```python
from build123d import *

# Parameters (mm, degrees)
SKETCH_2_W          = 1055.327979506
SKETCH_2_H          = 140
SKETCH_2_R          = 3
SKETCH_2_R_2        = 2.999999994
SKETCH_2_R_3        = 3.000000004
SKETCH_2_R_4        = 3.000000008
SKETCH_2_R_5        = 2.984817456
EXTRUDE_1_DEPTH     = 80
SKETCH_3_R          = 3
SKETCH_3_R_2        = 3.000000003
SKETCH_3_R_3        = 2.999999996
CUT_EXTRUDE_1_DEPTH = 10


with BuildPart() as part:
    # Эскиз2 → Бобышка-Вытянуть1 (new body)
    with BuildSketch(Plane(origin=(35, -236.577126762, 8.404450588), x_dir=(-1.3965925355372533e-14, -0.44721359549995804, -0.8944271909999159), z_dir=(2.4440369371901933e-14, -0.8944271909999159, 0.44721359549995804))):
        with Locations((247.509812295, 0)):
            Rectangle(SKETCH_2_W, SKETCH_2_H)
        with Locations((-220.154177458, 48.999999999)):
            Circle(SKETCH_2_R, mode=Mode.SUBTRACT)
        with Locations((-130.154177458, 49)):
            Circle(SKETCH_2_R, mode=Mode.SUBTRACT)
        with Locations((-220.154177458, -41.000000001)):
            Circle(SKETCH_2_R, mode=Mode.SUBTRACT)
        with Locations((-130.154177458, -41)):
            Circle(SKETCH_2_R, mode=Mode.SUBTRACT)
        with Locations((-40, 50)):
            Circle(SKETCH_2_R, mode=Mode.SUBTRACT)
        with Locations((-40, -40)):
            Circle(SKETCH_2_R, mode=Mode.SUBTRACT)
        with Locations((50, 50)):
            Circle(SKETCH_2_R, mode=Mode.SUBTRACT)
        with Locations((50, -40)):
            Circle(SKETCH_2_R, mode=Mode.SUBTRACT)
        with Locations((75, 50)):
            Circle(SKETCH_2_R, mode=Mode.SUBTRACT)
        with Locations((75, -40)):
            Circle(SKETCH_2_R, mode=Mode.SUBTRACT)
        with Locations((105, -57.5)):
            Circle(SKETCH_2_R, mode=Mode.SUBTRACT)
        with Locations((105, 35.5)):
            Circle(SKETCH_2_R, mode=Mode.SUBTRACT)
        with Locations((210, -57.5)):
            Circle(SKETCH_2_R, mode=Mode.SUBTRACT)
        with Locations((210, 35.5)):
            Circle(SKETCH_2_R, mode=Mode.SUBTRACT)
        with Locations((280, 50)):
            Circle(SKETCH_2_R, mode=Mode.SUBTRACT)
        with Locations((280, -41)):
            Circle(SKETCH_2_R, mode=Mode.SUBTRACT)
        with Locations((420, 50)):
            Circle(SKETCH_2_R, mode=Mode.SUBTRACT)
        with Locations((420, -40)):
            Circle(SKETCH_2_R, mode=Mode.SUBTRACT)
        with Locations((445, 50)):
            Circle(SKETCH_2_R, mode=Mode.SUBTRACT)
        with Locations((445, -40)):
            Circle(SKETCH_2_R, mode=Mode.SUBTRACT)
        with Locations((535, 50)):
            Circle(SKETCH_2_R, mode=Mode.SUBTRACT)
        with Locations((535, -40)):
            Circle(SKETCH_2_R, mode=Mode.SUBTRACT)
        with Locations((623.000000015, 49.999999971)):
            Circle(SKETCH_2_R_2, mode=Mode.SUBTRACT)
        with Locations((715.173802057, 50.999999957)):
            Circle(SKETCH_2_R_3, mode=Mode.SUBTRACT)
        with Locations((623, -40.000000029)):
            Circle(SKETCH_2_R_4, mode=Mode.SUBTRACT)
        with Locations((715.173802043, -39.000000043)):
            Circle(SKETCH_2_R, mode=Mode.SUBTRACT)
        with Locations((-57.5, -37.5)):
            Circle(SKETCH_2_R, mode=Mode.SUBTRACT)
        with Locations((-57.5, 47.5)):
            Circle(SKETCH_2_R, mode=Mode.SUBTRACT)
        with Locations((-112.5, 47.5)):
            Circle(SKETCH_2_R, mode=Mode.SUBTRACT)
        with Locations((-112.484817456, -37.5)):
            Circle(SKETCH_2_R_5, mode=Mode.SUBTRACT)
    extrude(amount=EXTRUDE_1_DEPTH)

    # Эскиз3 → Вырез-Вытянуть1 (cut)
    with BuildSketch(Plane(origin=(105, 0, 0), x_dir=(0, 0, -1), z_dir=(1, 0, 0))):
        with Locations((301.002749958, -418.113542766)):
            Circle(SKETCH_3_R)
        with Locations((289.375196475, -441.368649732)):
            Circle(SKETCH_3_R)
        with Locations((437.902966638, -469.334383556)):
            Circle(SKETCH_3_R)
        with Locations((559.545064612, -530.155432548)):
            Circle(SKETCH_3_R_2)
        with Locations((111.384185469, -323.304260514)):
            Circle(SKETCH_3_R_3)
        with Locations((99.756631986, -346.55936748)):
            Circle(SKETCH_3_R_3)
    extrude(amount=-CUT_EXTRUDE_1_DEPTH, mode=Mode.SUBTRACT)


solid = part.part
```
Work out the finished part from the listing and answer in its coordinate system (mm). Round coordinates to 2 decimals unless told otherwise and drop trailing zeros. Write each loop counter-clockwise with the first axis right and the second up, starting at its lowest first coordinate (ties: lowest second). Pieces come first, ordered by that corner, then holes.
1) Determine the mould class of faces 1 (the face through (34.02, -618.522, -667.294)), 2 (the face through (-4.325, -245.074, 79.601)), 3 (the face through (-5.87, -212.31, 145.14)), 4 (the face through (105, -379, -189)) for opening direction Y: pulls with the +Y half, pulls with the -Y half, needs draft (parallel to the pull), parting line crosses it, or undercut.
2) Consider probe 1 along Z at (x, y) = (-8, -162.5); probe 2 along Z at (x, y) = (-1, -190.5); probe 3 along Z at (x, y) = (39, -421). Determine where each line is inside the solid, lowest interval first.
3) A cutting plane is placed at B-B on z = -454.5. Give the number of separate pieces and of enclosed holes in the cut face, and give its area (3 significant figures).
4) Flat-ended cylindrical pins translate along their axes: P1, Ø3, axis at y = -531.5, z = -560, coming from the +X side; P2, Ø3, axis at y = -470.5, z = -439, coming from the +X side; P3, Ø5, axis at x = -8.5, z = -443, coming from the -Y side; P4, Ø2, axis at x = -13.5, y = -600.5, coming from the +Z side. Find the tip coordinate at first contact, or state that the pin passes through.
5) A cutting plane is placed at A-A on x = 24. Determine the outline of the cut face in (y, z).
Entries:
1. face 1: pulls with the -Y half
1. face 2: undercut
1. face 3: undercut
1. face 4: needs draft
2. probe 1: z = 156.56 to 215.01, 220.01 to 284.59
2. probe 2: z = 100.56 to 108.24, 114.01 to 279.44
2. probe 3: z = -360.44 to -181.56
3. separate pieces: 1
3. enclosed holes: 2
3. area: 12,400 mm2
4. P1: stops at x = 95
4. P2: stops at x = 105
4. P3: stops at y = -552.97
4. P4: stops at z = -538.56
5. outline: (-654.8, -649.15) - (-583.25, -684.93) - (-111.29, 258.98) - (-182.84, 294.76) - close
